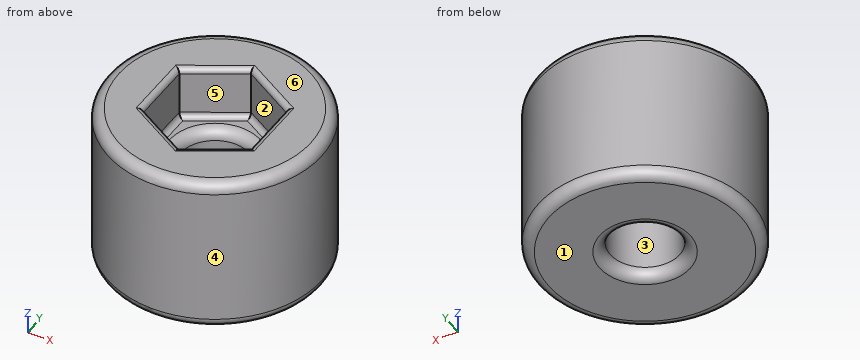
Autodesk Inventor part; units mm, degrees
ref_plane "YZ Plane" through (0, 0, 0) normal (1, 0, 0) x (0, 1, 0)
ref_plane "XZ Plane" through (0, 0, 0) normal (0, 1, 0) x (-1, 0, 0)
ref_plane "XY Plane" through (0, 0, 0) normal (0, 0, 1) x (1, 0, 0)
sketch "Sketch2" plane through (0, 0, 0) normal (0, 0, 1) x (1, 0, 0)
  circle A0 centre (0, 0) radius 10
  circle A1 centre (0, 0) radius 3.25
  dimension "d0" = 20
  dimension "d1" = 6.5
extrude "Extrusion1" add sketch "Sketch2" along normal blind 15
sketch "Sketch3" plane through (0, 0, 15) normal (0, 0, 1) x (1, 0, 0)
  circle A0 centre (0, 0) radius 3.25
  line L0 (5.0629, 2.8931) -> (5.037, -2.9381)
  line L1 (5.037, -2.9381) -> (-0.026, -5.8312)
  line L2 (-0.026, -5.8312) -> (-5.0629, -2.8931)
  line L3 (-5.0629, -2.8931) -> (-5.037, 2.9381)
  line L4 (-5.037, 2.9381) -> (0.026, 5.8312)
  line L5 (0.026, 5.8312) -> (5.0629, 2.8931)
  dimension "d4" = 10.1
extrude "Extrusion2" cut sketch "Sketch3" against normal blind 5
fillet "Fillet1" radius 0.5 12 edges at (-2.5055, 4.3846, 15) (2.5444, 4.3621, 15) (5.0499, -0.0225, 15) (2.5055, -4.3846, 15) (-2.5444, -4.3621, 15) (-5.0499, 0.0225, 15) (-5.0499, 0.0225, 10) (-2.5055, 4.3846, 10) (2.5444, 4.3621, 10) (5.0499, -0.0225, 10) (2.5055, -4.3846, 10) (-2.5444, -4.3621, 10)
fillet "Fillet2" radius 1 4 edges at (-3.25, 0, 10) (-3.25, 0, 0) (-10, 0, 15) (-10, 0, 0)
properties part number "ExtensionFastener"
Read the model definition and answer for the solid it produces. Units are mm, in the model's axes. Face numbers are marked on the shaded views. A direction names the side the tool comes from. Coordinates: 2 decimals unless noted, no trailing zeros. Write each loop counter-clockwise with the first axis right and the second up, starting at its lowest first coordinate (ties: lowest second). Pieces come first, ordered by that corner, then holes. Notation, with made-up numbers: (70, 54.5) -> (87, 54.5) arc R29 ccw to (87, 81.5) -> close; hole circle Ø2 at (6.25, 46.5). An arc over 180 degrees is marked (long way). Return JSON: item names as keys, results as strings.
1. Find the intervals of material crossed by line 1 along Y through (x, z) = (0, 5); line 2 along Y through (x, z) = (-2.25, 2.25); line 3 along X through (y, z) = (4, 8), in increasing order. Write a range as from..to.
Found:
{"line 1": "-10..-3.25, 3.25..10", "line 2": "-9.74..-2.35, 2.35..9.74", "line 3": "-9.17..9.17"}
2. Determine the mould class of the marked faces 3, 4, 5 and 6 for opening direction Y: pulls with the +Y half, pulls with the -Y half, needs draft (parallel to the pull), parting line crosses it, or undercut.
Found:
{"face 3": "undercut", "face 4": "parting line crosses it", "face 5": "undercut", "face 6": "needs draft"}
3. Each of these flat-tipped pins is pushed along its axis until it touches: P1, Ø3, axis at x = 6.5, z = 10.5, coming from the -Y side; P2, Ø2, axis at x = 2, z = 8, coming from the +Y side; P3, Ø4.5, axis at x = -1, y = -2, coming from the +Z side. Where does it stop, or does it pass through?
Found:
{"P1": "y = -8.66", "P2": "y = 9.95", "P3": "z = 10"}
4. A cutting plane is placed at A-A (z = 11). Determine the outline of the cut face in (x, y).
Found:
{"outline": "circle Ø20 at (0, 0); hole (-5.06, -2.89) -> (-0.03, -5.83) -> (5.04, -2.94) -> (5.06, 2.89) -> (0.03, 5.83) -> (-5.04, 2.94) -> close"}
5. A tool of negligible diameter and unlimited length cuts with its end or side. For the marked faces 1 and 2, from which of +Z, -Z, +X, -X, +Y, -Y can it reach the whole face along a straight path? Write none if from no direction.
Found:
{"face 1": "-Z, +X, -X, +Y, -Y", "face 2": "+Z"}
6. A cutting plane is placed at B-B (z = 6.75). Determine the outline of the cut face in (x, y), and give its area (3 significant figures).
Found:
{"outline": "circle Ø20 at (0, 0); hole circle Ø6.5 at (0, 0)", "area": "281 mm2"}
